Here's the drawing with two shaded views (mm, measured from the low corner). I have some questions. A direction names the side the tool comes from. Coordinates: 2 decimals unless noted, no trailing zeros. Loops run counter-clockwise (first coordinate to the right, second up) from the corner with the lowest first, then second, coordinate; pieces in that order, holes last. Notation, with made-up numbers: (59, 7.5) - (113, 7.5) arc R14 cw to (113, 27.5) - close; hole circle Ø11 at (50, -7). An arc over 180 degrees is marked (long way). Use a Markdown table: item, result.
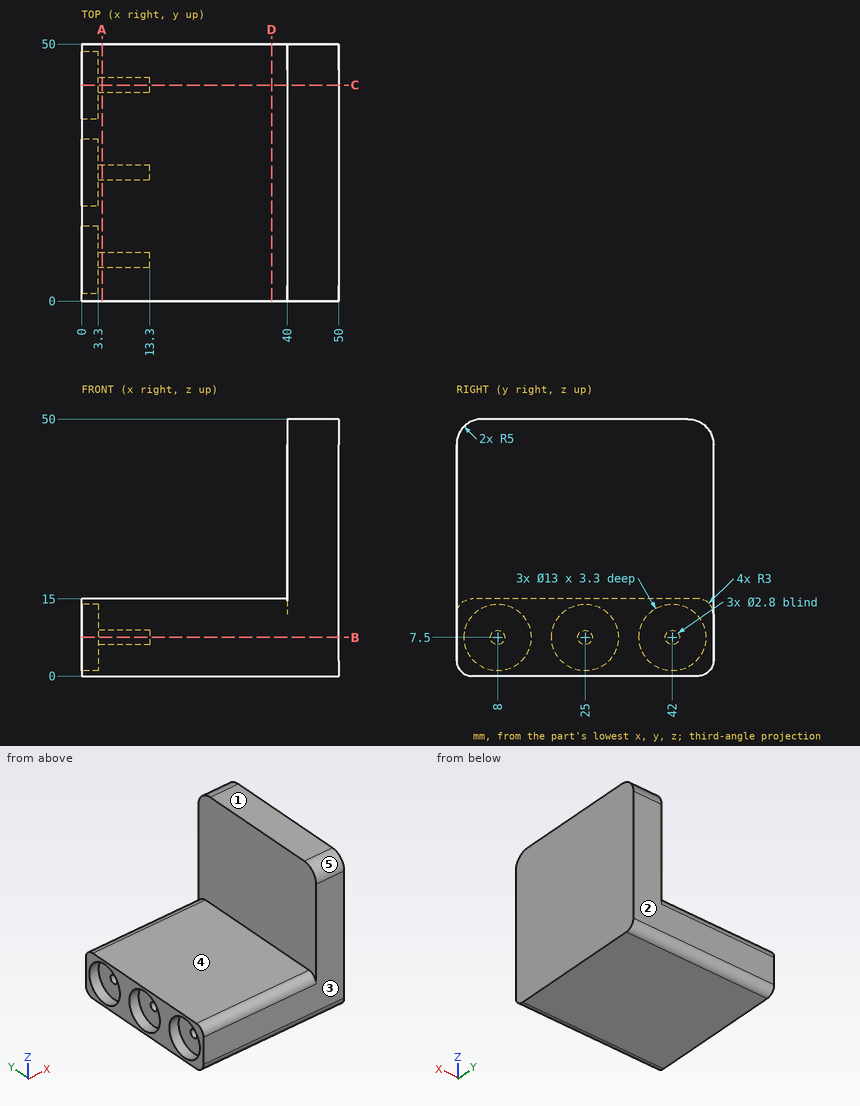
Q1. I want a section at C-C, the plane y = 42. Write out the boundary of the cut face in (x, z).
Check values:
| item | result |
|---|---|
| outline | (0, 0) - (50, 0) - (50, 50) - (40, 50) - (40, 15) - (0, 15) - (0, 14) - (3.3, 14) - (3.3, 8.9) - (13.3, 8.9) - (13.3, 6.1) - (3.3, 6.1) - (3.3, 1) - (0, 1) - close |
Q2. I want a section at D-D, the plane x = 37. Write out the boundary of the cut face in (y, z).
Check values:
| item | result |
|---|---|
| outline | (0, 3) arc R3 ccw to (3, 0) - (47, 0) arc R3 ccw to (50, 3) - (50, 12) arc R3 ccw to (47, 15) - (3, 15) arc R3 ccw to (0, 12) - close |
Q3. If we mould it in two halves opening along Y, with no side actions, what happens to the marked faces 1, 2 and 3? For each: pulls with the +Y half, pulls with the -Y half, needs draft (parallel to the pull), parting line crosses it, or undercut.
Check values:
| item | result |
|---|---|
| face 1 | needs draft |
| face 2 | pulls with the +Y half |
| face 3 | pulls with the -Y half |
Q4. I want a section at B-B, the plane z = 7.5. Write out the boundary of the cut face in (x, y), then the cut area to 3 significant figures.
Check values:
| item | result |
|---|---|
| outline | (0, 0) - (50, 0) - (50, 50) - (0, 50) - (0, 48.5) - (3.3, 48.5) - (3.3, 43.4) - (13.3, 43.4) - (13.3, 40.6) - (3.3, 40.6) - (3.3, 35.5) - (0, 35.5) - (0, 31.5) - (3.3, 31.5) - (3.3, 26.4) - (13.3, 26.4) - (13.3, 23.6) - (3.3, 23.6) - (3.3, 18.5) - (0, 18.5) - (0, 14.5) - (3.3, 14.5) - (3.3, 9.4) - (13.3, 9.4) - (13.3, 6.6) - (3.3, 6.6) - (3.3, 1.5) - (0, 1.5) - close |
| area | 2,290 mm^2 |
Q5. Please list where these lines run through material, in increasing order: L1, parallel to Z at x = 6.5, y = 25; L2, parallel to Z at x = 1, y = 8; L3, parallel to Y at x = 2, z = 7. Write a range as from..to.
Check values:
| item | result |
|---|---|
| L1 | 0..6.1, 8.9..15 |
| L2 | 0..1, 14..15 |
| L3 | 0..1.52, 14.48..18.52, 31.48..35.52, 48.48..50 |
Q6. Which directions (+Z, -Z, +X, -X, +Y, -Y) give clear straight access to the entire face, cutting with the end or side of a thin tool? Please do the marked faces 4 and 5.
Check values:
| item | result |
|---|---|
| face 4 | +Z, -X, +Y, -Y |
| face 5 | +Z, +X, -X, -Y |
Q7. Will these pins go through, and if not, where does the flat tip stop? P1, Ø2, axis at y = 25, z = 8, coming from the -X side; P2, Ø4, axis at y = 30, z = 36.5, coming from the -X side; P3, Ø12, axis at x = 16, y = 30.5, coming from the +Z side.
Check values:
| item | result |
|---|---|
| P1 | x = 3.3 |
| P2 | x = 40 |
| P3 | z = 15 |
Q8. I want a section at A-A, the plane x = 4. Write out the boundary of the cut face in (y, z).
Check values:
| item | result |
|---|---|
| outline | (0, 3) arc R3 ccw to (3, 0) - (47, 0) arc R3 ccw to (50, 3) - (50, 12) arc R3 ccw to (47, 15) - (3, 15) arc R3 ccw to (0, 12) - close; hole circle Ø2.8 at (8, 7.5); hole circle Ø2.8 at (25, 7.5); hole circle Ø2.8 at (42, 7.5) |
